Can you work these out from the model? Positions are in its coordinate system, mm. A direction names the side the tool comes from. Give positions to 0.01 mm unless a question says otherwise; leave off trailing zeros. Order: outer loops, then holes, each group sorted by start corner. A loop starts at its lowest first (then second) coordinate and runs counter-clockwise, first axis right, second up.
Autodesk Inventor part; units mm, degrees
ref_plane "holder_XY" through (0, 0, 0) normal (0, 0, 1) x (1, 0, 0)
ref_plane "holder_YZ" through (0, 0, 0) normal (1, 0, 0) x (0, 1, 0)
ref_plane "holder_ZX" through (0, 0, 0) normal (0, 1, 0) x (0, 0, 1)
sketch "Sketch_1" plane through (0, 0, 0) normal (0, 0, 1) x (1, 0, 0)
  line L0 (28, 0) -> (-4.0667, 0)
  line L1 (13, 0) -> (13, 1.5)
  line L2 (13, 1.5) -> (6.1703, 1.5)
  arc A0 (6.1703, 1.5) -> (-4.0667, 4.877) centre (0, 0) ccw
  line L3 (-4.0667, 4.877) -> (-4.0667, 10)
  line L4 (-4.0667, 10) -> (0, 10)
  arc A1 (13, 5) -> (0, 10) centre (-2.0333, -14.6867) ccw
  line L5 (13, 5) -> (23, 5)
  line L6 (23, 5) -> (23, 5.5)
  line L7 (23, 5.5) -> (24, 6.5)
  line L8 (24, 6.5) -> (27.35, 6.5)
  arc A2 (28, 5.85) -> (27.35, 6.5) centre (27.35, 5.85) ccw
  line L9 (28, 5.85) -> (28, 0)
  line L10 (28, 0) -> (13, 0)
revolve "Revolution1" add sketch "Sketch_1" angle 360 about axis through (28, 0, 0) along (1, 0, 0)
sketch "Sketch_2" plane through (28, 0, 0) normal (1, 0, 0) x (0, 0, -1)
  line L0 (-22, 26) -> (-22, -26)
  line L1 (-22, -26) -> (22, -26)
  line L2 (22, -26) -> (22, 26)
  line L3 (22, 26) -> (-22, 26)
  line L4 (-5.5, 13) -> (-5.5, -13)
  line L5 (-5.5, -13) -> (5.5, -13)
  line L6 (5.5, -13) -> (5.5, 13)
  line L7 (5.5, 13) -> (-5.5, 13)
extrude "Extrusion1" cut sketch "Sketch_2" against normal blind 5
sketch "Sketch_6" plane through (0, 0, 0) normal (0, 0, 1) x (1, 0, 0)
  line L0 (-2.0333, 0) -> (-8.1333, 0)
  arc A0 (-5.6933, 10) -> (-6.0214, 5.1422) centre (-5.6933, 7.56) ccw
  line L1 (-6.0214, 5.1422) -> (-4.0667, 4.877)
  arc A1 (-2.0333, 6.0157) -> (-4.0667, 4.877) centre (0, 0) ccw
  line L2 (-2.0333, 6.0157) -> (-2.0333, 10)
  line L3 (-2.0333, 10) -> (-5.6933, 10)
revolve "Revolution2" add sketch "Sketch_6" angle 360 about axis through (-2.0333, 0, 0) along (1, 0, 0)
sketch "Sketch4" plane through (28, -1.9931, -5.5) normal (1, 0, 0) x (0, 0, -1)
  point P0 (-5.5, 1.9931)
hole "Hole1" at (28, 0, 0) direction (-1, 0, 0) diameter 4.917 depth 16.5806 tip angle 120 countersink diameter 6 countersink angle 90
ref_plane "holder_XY" through (0, 0, 0) normal (0, 0, 1) x (1, 0, 0)
ref_plane "holder_YZ" through (0, 0, 0) normal (1, 0, 0) x (0, 1, 0)
ref_plane "holder_ZX" through (0, 0, 0) normal (0, 1, 0) x (0, 0, 1)
properties part number "RBID6holder"
1) I'm going to push flat-ended pins straight in: pin 1 Ø1 at (x, z) = (14, 6) entering from +Y; pin 2 Ø12 at (x, y) = (-0.5, 6) entering from -Z; pin 3 Ø2 at (y, z) = (5.5, 7.5) entering from +X; pin 4 Ø4 at (y, z) = (8, -0.5) entering from +X. Where does each tip first touch, or does it pass through?
2) Which directions (+Z, -Z, +X, -X, +Y, -Y) give clear straight access to the entire face, cutting with the end or side of a thin tool? Please do faces 4 (the face through (26, 0, 5.5)), 5 (the face through (25.7, 6.5, -0.1)), 6 (the face through (23, 1.6, -4.9)), 7 (the face through (19.327, -0.738, -2.345)), 8 (the face through (23.2, 5.7, -0.1)).
3) We'd pull the mould along X, two halves only. Please class faces 1 (the face through (23.2, -5.7, 0.1)), 2 (the face through (28, 3, -2)), 3 (the face through (-4.41, 2.27, 4.37)): +X half, -X half, draft (parallel to the pull), parting line (faces both ways), or undercut.
4) If I drill on line 1 (Z direction, x = 20, y = 0); line 2 (Y direction, x = 9.9, z = 0); line 3 (Y direction, x = 18.5, z = -1), over which ranges is the centre line in solid material (lowest first)?
5) Suppose I cut it at A-A (x = 22.5). Please give me the cut outline in (y, z), and give its area (3 significant figures).
Results:
1. pin 1: passes through
1. pin 2: stops at z = -10
1. pin 3: stops at x = 7.19
1. pin 4: stops at x = 27.98
2. face 4: +Z, +X, +Y, -Y
2. face 5: +X, +Y
2. face 6: none
2. face 7: +X
2. face 8: +Y
3. face 1: undercut
3. face 2: +X half
3. face 3: -X half
4. line 1: z = -5 to -2.46, 2.46 to 5
4. line 2: y = -7.02 to -1.5, 1.5 to 7.02
4. line 3: y = -4.9 to -2.25, 2.25 to 4.9
5. outline: circle Ø10 at (0, 0); hole circle Ø4.92 at (0, 0)
5. area: 59.6 mm2
